Can you work these out from the model? Positions are in its coordinate system, mm. Round coordinates to 2 decimals unless told otherwise and drop trailing zeros. One line per question, with ' | ' between items.
```python
from build123d import *

# Parameters (mm, degrees)
SKETCH1_R                            = 4.35
BOSS_EXTRUDE1_DEPTH                  = 8
SKETCH2_R                            = 11
SKETCH2_R_2                          = 4.35
BOSS_EXTRUDE2_DEPTH                  = 1
SKETCH3_R                            = 8.3
SKETCH3_R_2                          = 4.35
BOSS_EXTRUDE3_DEPTH                  = 6
SZKIC9_OUTSIDE_W                     = 34.824
SZKIC9_OUTSIDE_H                     = 38.228
SZKIC9_OUTSIDE_R                     = 11
WYTNIJ_WYCI_GNI_CIE3_DEPTH           = 1
WYTNIJ_WYCI_GNI_CIE3_DRAFT           = -60
SZKIC10_OUTSIDE_W                    = 34.824
SZKIC10_OUTSIDE_H                    = 38.228
SZKIC10_OUTSIDE_R                    = 11
WYTNIJ_WYCI_GNI_CIE4_DEPTH           = 1
WYTNIJ_WYCI_GNI_CIE4_DRAFT           = -60
SZKIC11_R                            = 5.35
WYTNIJ_WYCI_GNI_CIE5_DEPTH           = 1
WYTNIJ_WYCI_GNI_CIE5_DRAFT           = -60
SZKIC13_OUTSIDE_W                    = 33.36
SZKIC13_OUTSIDE_H                    = 36.764
SZKIC13_OUTSIDE_R                    = 7.3
WYTNIJ_WYCI_GNI_CIE8_DEPTH           = 1
WYTNIJ_WYCI_GNI_CIE8_DRAFT           = -45
SZKIC13_OUTSIDE_R_2                  = 5.35
WYTNIJ_WYCI_GNI_CIE8_PROFILE_2_DEPTH = 1
WYTNIJ_WYCI_GNI_CIE8_PROFILE_2_DRAFT = -45


with BuildPart() as part:
    # Sketch1 → Boss-Extrude1 (new body)
    with BuildSketch(Plane.XY):
        Polygon((-11, 6.350852961), (-11, -6.350852961), (0, -12.701705922), (11, -6.350852961), (11, 6.350852961), (0, 12.701705922), align=None)
        Circle(SKETCH1_R, mode=Mode.SUBTRACT)
    extrude(amount=BOSS_EXTRUDE1_DEPTH)

    # Sketch2 → Boss-Extrude2 (add)
    with BuildSketch(Plane.XY.offset(8)):
        Circle(SKETCH2_R)
        Circle(SKETCH2_R_2, mode=Mode.SUBTRACT)
    extrude(amount=BOSS_EXTRUDE2_DEPTH)

    # Sketch3 → Boss-Extrude3 (add)
    with BuildSketch(Plane.XY.offset(9)):
        Circle(SKETCH3_R)
        Circle(SKETCH3_R_2, mode=Mode.SUBTRACT)
    extrude(amount=BOSS_EXTRUDE3_DEPTH)


with BuildPart() as wytnij_wyci_gni_cie3_tool:
    # Szkic9 outside → Wytnij-wyciągnięcie3 (with draft: the straight prism first)
    with BuildSketch(Plane(origin=(0, 0, 0), x_dir=(-1, 0, 0), z_dir=(0, 0, -1))):
        Rectangle(SZKIC9_OUTSIDE_W, SZKIC9_OUTSIDE_H)
        with Locations(Location((0, 0, 0), (0, 0, 180))):
            Circle(SZKIC9_OUTSIDE_R, mode=Mode.SUBTRACT)
    extrude(amount=-WYTNIJ_WYCI_GNI_CIE3_DEPTH)
    # Wytnij-wyciągnięcie3: the draft: its side faces are tilted about the plane it starts from
    wytnij_wyci_gni_cie3_sides = [wytnij_wyci_gni_cie3_tool.faces().sort_by_distance(p)[0] for p in [
        (0, -19.114, 0.5),
        (-17.412, 0, 0.5),
        (0, 19.114, 0.5),
        (17.412, 0, 0.5),
        (-11, 0, 0.5),
    ]]
    draft(wytnij_wyci_gni_cie3_sides, Plane(origin=(0, 0, 0), x_dir=(-1, 0, 0), z_dir=(0, 0, -1)), WYTNIJ_WYCI_GNI_CIE3_DRAFT)


with BuildPart() as part_1:
    add(part.part)

    # Wytnij-wyciągnięcie3: cut by wytnij_wyci_gni_cie3_tool
    add(wytnij_wyci_gni_cie3_tool.part, mode=Mode.SUBTRACT)


with BuildPart() as wytnij_wyci_gni_cie4_tool:
    # Szkic10 outside → Wytnij-wyciągnięcie4 (with draft: the straight prism first)
    with BuildSketch(Plane.XY.offset(8)):
        Rectangle(SZKIC10_OUTSIDE_W, SZKIC10_OUTSIDE_H)
        Circle(SZKIC10_OUTSIDE_R, mode=Mode.SUBTRACT)
    extrude(amount=-WYTNIJ_WYCI_GNI_CIE4_DEPTH)
    # Wytnij-wyciągnięcie4: the draft: its side faces are tilted about the plane it starts from
    wytnij_wyci_gni_cie4_sides = [wytnij_wyci_gni_cie4_tool.faces().sort_by_distance(p)[0] for p in [
        (0, -19.114, 7.5),
        (17.412, 0, 7.5),
        (0, 19.114, 7.5),
        (-17.412, 0, 7.5),
        (-11, 0, 7.5),
    ]]
    draft(wytnij_wyci_gni_cie4_sides, Plane.XY.offset(8), WYTNIJ_WYCI_GNI_CIE4_DRAFT)


with BuildPart() as part_2:
    add(part_1.part)

    # Wytnij-wyciągnięcie4: cut by wytnij_wyci_gni_cie4_tool
    add(wytnij_wyci_gni_cie4_tool.part, mode=Mode.SUBTRACT)


with BuildPart() as wytnij_wyci_gni_cie5_tool:
    # Szkic11 → Wytnij-wyciągnięcie5 (with draft: the straight prism first)
    with BuildSketch(Plane(origin=(0, 0, 0), x_dir=(-1, 0, 0), z_dir=(0, 0, -1))):
        Circle(SZKIC11_R)
    extrude(amount=-WYTNIJ_WYCI_GNI_CIE5_DEPTH)
    # Wytnij-wyciągnięcie5: the draft: its side faces are tilted about the plane it starts from
    wytnij_wyci_gni_cie5_sides = [wytnij_wyci_gni_cie5_tool.faces().sort_by_distance(p)[0] for p in [
        (5.35, 0, 0.5),
    ]]
    draft(wytnij_wyci_gni_cie5_sides, Plane(origin=(0, 0, 0), x_dir=(-1, 0, 0), z_dir=(0, 0, -1)), WYTNIJ_WYCI_GNI_CIE5_DRAFT)


with BuildPart() as part_3:
    add(part_2.part)

    # Wytnij-wyciągnięcie5: cut by wytnij_wyci_gni_cie5_tool
    add(wytnij_wyci_gni_cie5_tool.part, mode=Mode.SUBTRACT)


with BuildPart() as wytnij_wyci_gni_cie8_tool:
    # Szkic13 outside → Wytnij-wyciągnięcie8 (with draft: the straight prism first)
    with BuildSketch(Plane.XY.offset(15)):
        Rectangle(SZKIC13_OUTSIDE_W, SZKIC13_OUTSIDE_H)
        Circle(SZKIC13_OUTSIDE_R, mode=Mode.SUBTRACT)
    extrude(amount=-WYTNIJ_WYCI_GNI_CIE8_DEPTH)
    # Wytnij-wyciągnięcie8: the draft: its side faces are tilted about the plane it starts from
    wytnij_wyci_gni_cie8_sides = [wytnij_wyci_gni_cie8_tool.faces().sort_by_distance(p)[0] for p in [
        (0, -18.382, 14.5),
        (16.68, 0, 14.5),
        (0, 18.382, 14.5),
        (-16.68, 0, 14.5),
        (-7.3, 0, 14.5),
    ]]
    draft(wytnij_wyci_gni_cie8_sides, Plane.XY.offset(15), WYTNIJ_WYCI_GNI_CIE8_DRAFT)


with BuildPart() as part_4:
    add(part_3.part)

    # Wytnij-wyciągnięcie8: cut by wytnij_wyci_gni_cie8_tool
    add(wytnij_wyci_gni_cie8_tool.part, mode=Mode.SUBTRACT)


with BuildPart() as wytnij_wyci_gni_cie8_profile_2_tool:
    # Szkic13 outside → Wytnij-wyciągnięcie8 profile 2 (with draft: the straight prism first)
    with BuildSketch(Plane.XY.offset(15)):
        Circle(SZKIC13_OUTSIDE_R_2)
    extrude(amount=-WYTNIJ_WYCI_GNI_CIE8_PROFILE_2_DEPTH)
    # Wytnij-wyciągnięcie8 profile 2: the draft: its side faces are tilted about the plane it starts from
    wytnij_wyci_gni_cie8_profile_2_sides = [wytnij_wyci_gni_cie8_profile_2_tool.faces().sort_by_distance(p)[0] for p in [
        (-5.35, 0, 14.5),
    ]]
    draft(wytnij_wyci_gni_cie8_profile_2_sides, Plane.XY.offset(15), WYTNIJ_WYCI_GNI_CIE8_PROFILE_2_DRAFT)


with BuildPart() as part_5:
    add(part_4.part)

    # Wytnij-wyciągnięcie8 profile 2: cut by wytnij_wyci_gni_cie8_profile_2_tool
    add(wytnij_wyci_gni_cie8_profile_2_tool.part, mode=Mode.SUBTRACT)


solid = part_5.part
```
(1) Will these pins go through, and if not, where does the flat tip stop? pin 1 Ø4 at (x, z) = (7.5, 2.5) entering from -Y; pin 2 Ø2 at (x, z) = (7.5, 1.5) entering from +Y; pin 3 Ø8 at (x, y) = (0, 0) entering from -Z; pin 4 Ø2 at (x, z) = (-2.5, 8.5) entering from +Y.
Final values:
pin 1: y = -9.53 | pin 2: y = 8.95 | pin 3: through | pin 4: y = 11.51
(2) Please list where these lines run through material, in increasing order: probe 1 along Y at (x, z) = (0, 10.75); probe 2 along X at (y, z) = (0, 8.5); probe 3 along Z at (x, y) = (9, -3.5). Write a range as [from, to].
Final values:
probe 1: [-8.3, -4.35], [4.35, 8.3] | probe 2: [-11, -4.35], [4.35, 11] | probe 3: [0, 9]
(3) Thinking about a two-plate mould opening in X: for faces 1 (the conical face through (-9.864, -5.727, 0.234)), 2 (the cylindrical face through (-0.943, -4.247, 7.195)), 3 (the flat face through (4, 4, 15)), 4 (the cylindrical face through (-2.38, -10.74, 8.49)), which applies, released by +X, released by -X, zero draft, split by the parting line, or undercut?
Final values:
face 1: released by -X | face 2: undercut | face 3: zero draft | face 4: split by the parting line
